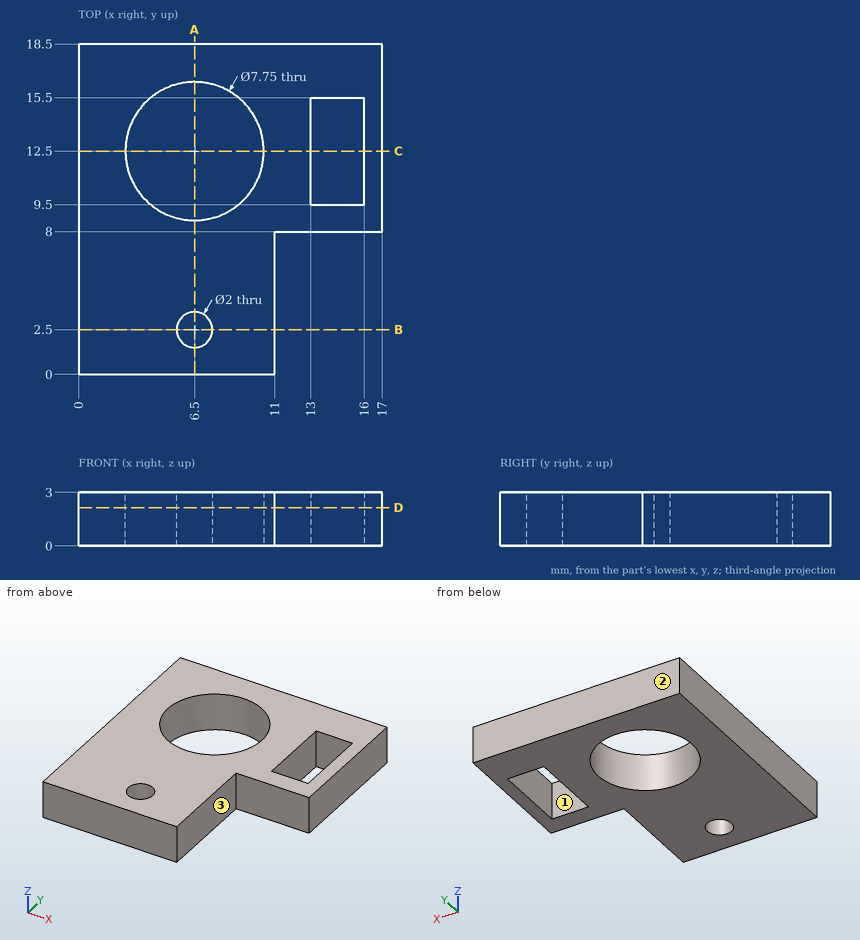
Geometry check sheet. Reference: drawing and pictorial views, mm from the part's lowest x, y, z. A direction names the side the tool comes from. Give positions to 0.01 mm unless a question says otherwise; leave off trailing zeros. Order: outer loops, then holes, each group sorted by start corner. A loop starts at its lowest first (then second) coordinate and runs counter-clockwise, first axis right, second up. Notation, with made-up numbers: M 51.25,41 L 57.25,41 A23 ccw 57.25,58 Z; hole C 3.5,49.5 d5. An arc over 180 degrees is marked long. Answer in a Markdown table with one row per item. Add a question column.
Item 1: Scan lines: probe 1 along Y at (x, z) = (6.5, 1.35) (3 decimals); probe 2 along Y at (x, z) = (14.75, 0.95); probe 3 along X at (y, z) = (5.25, 0.4). Record each from-to range of solid material in increasing order. Write a range as from..to.
Item 2: Tool access check on the marked faces 1, 2 and 3. Record the directions out of +Z, -Z, +X, -X, +Y, -Y that give a thin tool (end or side, any length) a straight path to the whole face; none if there is none.
Item 3: Section check D-D, the plane z = 2.15. Enter the section's corners in (x, y) (3 decimals).
Item 4: Section check C-C, the plane y = 12.5. Enter the section's corners in (x, z) (3 decimals), and give its area (4 significant figures).
Item 5: Gauge pin test, flat end, axial feed: pin 1 (1.5 mm diameter, centred on x = 14, z = 2, fed in from -Y). Record the tip position at first contact, or that the pin passes through.
Item 6: Section check B-B, the plane y = 2.5. Enter the section's corners in (x, z), and give its area (3 significant figures).
Item 7: Section check A-A, the plane x = 6.5. Enter the section's corners in (y, z) (3 decimals), and give its area (4 significant figures).
Filled sheet:
| question | item | result |
|---|---|---|
| 1 | probe 1 | y = 0..1.5, 3.5..8.625, 16.375..18.5 |
| 1 | probe 2 | y = 8..9.5, 15.5..18.5 |
| 1 | probe 3 | x = 0..11 |
| 2 | face 1 | +Z, -Z |
| 2 | face 2 | +Z, -Z, +X, -X, +Y |
| 2 | face 3 | +Z, -Z, +X, -Y |
| 3 | outline | M 0,0 L 11,0 L 11,8 L 17,8 L 17,18.5 L 0,18.5 Z; hole C 6.5,12.5 d7.75; hole C 6.5,2.5 d2; hole M 13,9.5 L 16,9.5 L 16,15.5 L 13,15.5 Z |
| 4 | outline | M 0,0 L 2.625,0 L 2.625,3 L 0,3 Z; M 10.375,0 L 13,0 L 13,3 L 10.375,3 Z; M 16,0 L 17,0 L 17,3 L 16,3 Z |
| 4 | area | 18.75 mm^2 |
| 5 | pin 1 | stops at y = 8 |
| 6 | outline | M 0,0 L 5.5,0 L 5.5,3 L 0,3 Z; M 7.5,0 L 11,0 L 11,3 L 7.5,3 Z |
| 6 | area | 27.0 mm^2 |
| 7 | outline | M 0,0 L 1.5,0 L 1.5,3 L 0,3 Z; M 3.5,0 L 8.625,0 L 8.625,3 L 3.5,3 Z; M 16.375,0 L 18.5,0 L 18.5,3 L 16.375,3 Z |
| 7 | area | 26.25 mm^2 |
